Verification items for this drawing (mm, ordinates from the low corner). A direction names the side the tool comes from. Round coordinates to 2 decimals unless told otherwise and drop trailing zeros. Order: outer loops, then holes, each group sorted by start corner. A loop starts at its lowest first (then second) coordinate and runs counter-clockwise, first axis right, second up. Notation, with made-up numbers: (65, 14) -> (86, 14) arc R15 ccw to (86, 33) -> close; hole circle Ø2 at (13, 55.5). An arc over 180 degrees is marked (long way). Answer in a Markdown table with one row per item. Add a question column.
1. Sectioned sample at B-B, the plane y = 4. Record the boundary of the cut face in (x, z), then the cut area to 3 significant figures.
2. Sectioned sample at D-D, the plane y = 2. Record the boundary of the cut face in (x, z).
3. Depth check by flat-ended pin: P1, Ø4, axis at x = 28, y = 6.5, coming from the -Z side; P2, Ø13.5, axis at x = 20.25, z = 13.25, coming from the +Y side; P3, Ø3, axis at y = 2, z = 4, coming from the -X side; P4, Ø4, axis at x = 10.5, y = 1.5, coming from the +Z side. Enter the tip coordinate at first touch or a pass-through.
4. Sectioned sample at A-A, the plane x = 20.25. Record the boundary of the cut face in (y, z).
5. Draft check along X on the marked faces 4, 5, 6 and 7. Enter one of: +X half, -X half, draft (parallel to the pull), parting line (faces both ways), or undercut.
6. Access from +Z, -Z, +X, -X, +Y, -Y to the whole of each face (thin tool, end or side, straight path). Record for the marked faces 1, 2 and 3.
7. Material ranges on L1, parallel to Z at x = 20.25, y = 4; L2, parallel to X at y = 3.25, z = 7.5; L3, parallel to Z at x = 16, y = 2, recorded low to high. Write a range as from..to.
8. Sectioned sample at C-C, the plane z = 19.75. Record the boundary of the cut face in (x, y).
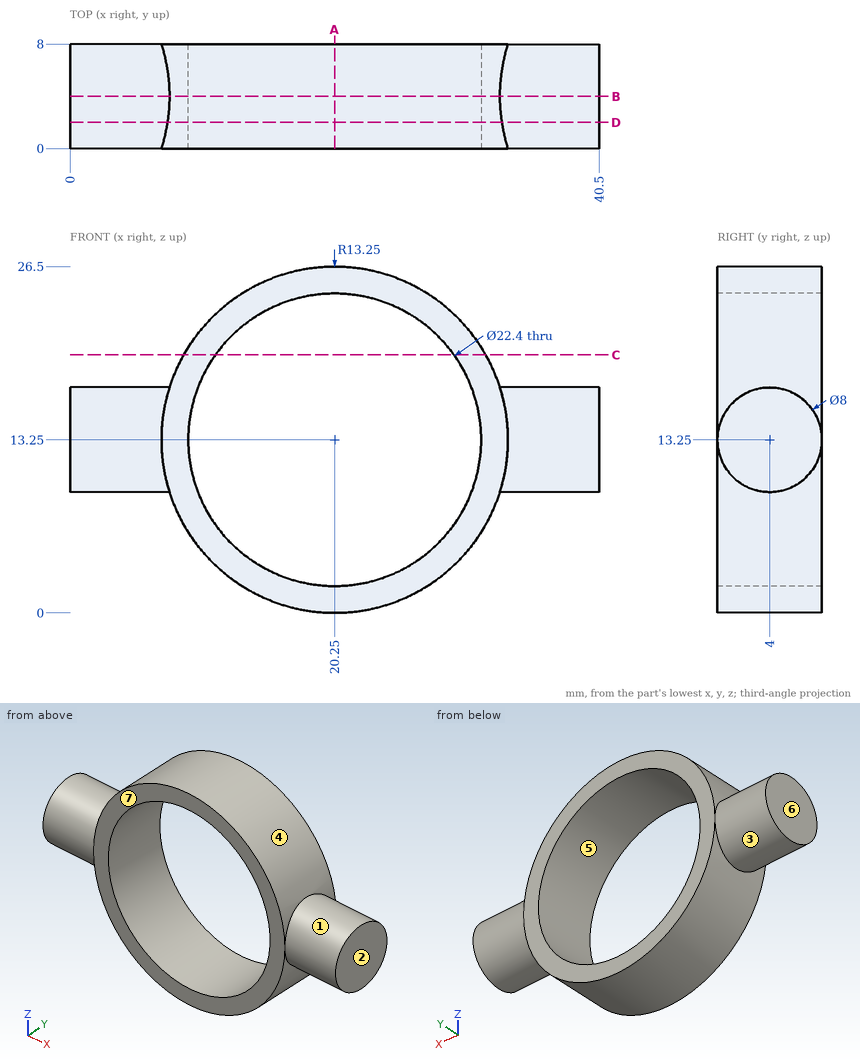
Answer key:
| question | item | result |
|---|---|---|
| 1 | outline | (0, 9.25) -> (7.62, 9.25) arc R13.25 ccw to (32.88, 9.25) -> (40.5, 9.25) -> (40.5, 17.25) -> (32.88, 17.25) arc R13.25 ccw to (7.62, 17.25) -> (0, 17.25) -> close; hole circle Ø22.4 at (20.25, 13.25) |
| 1 | area | 273 mm² |
| 2 | outline | (0, 9.79) -> (7.46, 9.79) arc R13.25 ccw to (33.04, 9.79) -> (40.5, 9.79) -> (40.5, 16.71) -> (33.04, 16.71) arc R13.25 ccw to (7.46, 16.71) -> (0, 16.71) -> close; hole circle Ø22.4 at (20.25, 13.25) |
| 3 | P1 | stops at z = 1.31 |
| 3 | P2 | passes through |
| 3 | P3 | stops at x = 9.5 |
| 3 | P4 | stops at z = 24 |
| 4 | outline | (0, 0) -> (8, 0) -> (8, 2.05) -> (0, 2.05) -> close; (0, 24.45) -> (8, 24.45) -> (8, 26.5) -> (0, 26.5) -> close |
| 5 | face 4 | parting line |
| 5 | face 5 | undercut |
| 5 | face 6 | -X half |
| 5 | face 7 | draft |
| 6 | face 1 | +X |
| 6 | face 2 | +Z, -Z, +X, +Y, -Y |
| 6 | face 3 | -X |
| 7 | L1 | z = 0..2.05, 24.45..26.5 |
| 7 | L2 | x = 8.31..10.64, 29.86..32.19 |
| 7 | L3 | z = 0.7..2.89, 23.61..25.8 |
| 8 | outline | (8.7, 0) -> (11.13, 0) -> (11.13, 8) -> (8.7, 8) -> close; (29.37, 0) -> (31.8, 0) -> (31.8, 8) -> (29.37, 8) -> close |
